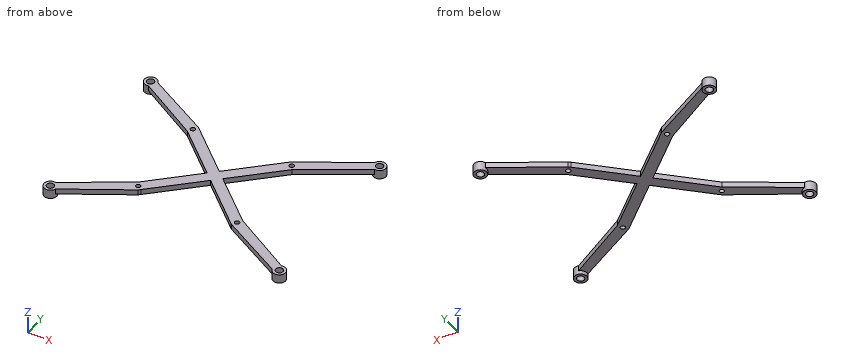
Autodesk Fusion 360 part; units mm, degrees
sketch "Sketch1" plane through (0, 0, 0) normal (0, 0, 1) x (1, 0, 0)
  line L0 (0, 0) -> (126.2, 0) construction
  line L1 (126.2, 0) -> (126.2, 92.7) construction
  line L2 (126.2, 92.7) -> (0, 92.7) construction
  line L3 (0, 92.7) -> (0, 0) construction
  circle A0 centre (126.2, 0) radius 2
  circle A1 centre (126.2, 92.7) radius 2
  circle A2 centre (0, 92.7) radius 2
  circle A3 centre (0, 0) radius 2
  line L4 (0, 92.7) -> (-5, 92.7) construction
  line L5 (0, 92.7) -> (0, 97.7) construction
  line L6 (0, 97.7) -> (-5, 92.7) construction
  line L7 (126.2, 0) -> (131.2, 0) construction
  line L8 (126.2, 0) -> (126.2, -5) construction
  line L9 (126.2, -5) -> (131.2, 0) construction
  line L10 (-2.5, 95.2) -> (128.7, 95.2)
  line L11 (128.7, 95.2) -> (128.7, -2.5)
  line L12 (128.7, -2.5) -> (-2.5, -2.5)
  line L13 (-2.5, -2.5) -> (-2.5, 95.2)
  line L14 (35.8499, 71.5999) -> (90.3499, 71.5999) construction
  line L15 (90.3499, 71.5999) -> (90.3499, 21.0999) construction
  line L16 (90.3499, 21.0999) -> (35.8499, 21.0999) construction
  line L17 (35.8499, 21.0999) -> (35.8499, 71.5999) construction
  line L18 (126.2, 0) -> (0, 92.7) construction
  line L19 (126.2, 92.7) -> (0, 0) construction
  line L20 (35.8499, 71.5999) -> (90.3499, 21.0999) construction
  line L21 (90.3499, 71.5999) -> (35.8499, 21.0999) construction
  circle A4 centre (35.8499, 71.5999) radius 1.3
  circle A5 centre (90.3499, 71.5999) radius 1.3
  circle A6 centre (90.3499, 21.0999) radius 1.3
  circle A7 centre (35.8499, 21.0999) radius 1.3
  circle A8 centre (90.3499, 71.5999) radius 3
  circle A9 centre (35.8499, 71.5999) radius 3
  circle A10 centre (35.8499, 21.0999) radius 3
  circle A11 centre (90.3499, 21.0999) radius 3
  circle A12 centre (126.2, 0) radius 2.5
  circle A13 centre (126.2, 92.7) radius 2.5
  circle A14 centre (0, 92.7) radius 2.5
  circle A15 centre (0, 0) radius 2.5
  line L22 (-1.5, 2) -> (34.2965, 23.6664)
  line L23 (1.5, -2) -> (37.3392, 18.4957)
  line L24 (91.9033, 23.6664) -> (127.4939, 2.1391)
  line L25 (88.8606, 18.4957) -> (124.7009, -2.0006)
  line L26 (37.3392, 74.2041) -> (1.5012, 94.6991)
  line L27 (34.2965, 69.0334) -> (-1.2939, 90.5609)
  line L28 (91.9033, 69.0334) -> (127.4939, 90.5609)
  line L29 (88.8606, 74.2041) -> (124.6996, 94.6997)
  line L30 (37.3392, 18.4957) -> (91.9033, 69.0334)
  line L31 (34.2965, 23.6664) -> (88.8606, 74.2041)
  line L32 (34.2965, 69.0334) -> (88.309, 18.9011)
  line L33 (91.9033, 23.6664) -> (37.3392, 74.2041)
  circle A16 centre (0, 92.7) radius 3.5
  circle A17 centre (0, 0) radius 3.5
  circle A18 centre (126.2, 0) radius 3.5
  circle A19 centre (126.2, 92.7) radius 3.5
  point P0 (-2.5, 95.2)
  point P1 (128.7, -2.5)
  dimension "d1" = 126.2
  dimension "d2" = 92.7
  dimension "d3" = 4
  dimension "d4" = 4
  dimension "d5" = 4
  dimension "d6" = 4
  dimension "d7" = 5
  dimension "d8" = 5
  dimension "d9" = 5
  dimension "d10" = 5
  dimension "d11" = 54.5
  dimension "d12" = 50.5
  dimension "d13" = 2.6
  dimension "d14" = 2.6
  dimension "d15" = 2.6
  dimension "d16" = 2.6
  dimension "d17" = 6
  dimension "d18" = 6
  dimension "d19" = 6
  dimension "d20" = 6
  dimension "d25" = 7
  dimension "d26" = 7
  dimension "d27" = 7
  dimension "d28" = 7
extrude "Extrude1" add sketch "Sketch1" along normal blind 3 contours A14 | A14 L26 L27 A16 | A9 L26 L27 A16 | A13 | A8 L28 L29 A19 | A13 L28 L29 A19 | A9 L33 | A15 L22 | A15 L22 L23 A17 | A10 L22 L23 A17 | A9 L31 L32 L33 | A8 L31 | A10 L30 L31 L32 | A10 L30 | L30 L31 L32 L33 | A8 L30 L31 L33 | A11 L30 L32 L33 | A11 | A12 | A11 L24 L25 A18 | A12 L24 L25 A18 picked at (37.444, 73.3682) picked at (-1.1921, 1.9962) picked at (88.7557, 73.3682) picked at (37.444, 19.3316)
extrude "Extrude2" add sketch "Sketch1" along normal blind -2 and the other way blind -3 contours L10 A16 | L10 L13 A14 A16 | L13 A16 | L10 A14 L26 A16 | A14 | L13 A14 L27 A16 | A14 L26 L27 A16 | L10 A19 | L10 A13 L29 A19 | L13 A15 L22 A17 | L13 A17 | L10 L11 A13 A19 | A13 | A13 L28 L29 A19 | L12 L13 A15 A17 | A15 L22 | A15 L22 L23 A17 | L11 A19 | L11 A13 L28 A19 | L12 A15 L23 A17 | L12 A17 | L11 A18 | L11 A12 L24 A18 | L12 A12 L25 A18 | L12 A18 | A12 | L11 L12 A12 A18 | A12 L24 L25 A18 picked at (-1.1921, 1.9962)
thread "Thread1"
Part model, mm, in its own coordinate system. Round coordinates to 2 decimals unless told otherwise and drop trailing zeros. Order: outer loops, then holes, each group sorted by start corner. A loop starts at its lowest first (then second) coordinate and runs counter-clockwise, first axis right, second up. Notation, with made-up numbers: M 17.25,2.25 L 43.25,2.25 A31 cw 43.25,35.25 Z; hole C -16.5,8 d3. An arc over 180 degrees is marked long. Answer in a Markdown table with one row per item. Add a question column.
Q1. Wall check: L1, parallel to Y at x = 0, z = -0.5; L2, parallel to X at y = 1, z = -1.5; L3, parallel to Z at x = 42.5, y = 23.5. Give the ranges that are in metal, low to high. Write a range as from..to.
Q2. Cut at A-A on y = 13. Give the cut face in (x, z), and give its area (3 significant figures).
Q3. Pin check, flat tips, straight feed: pin 1 (2 mm diameter, centred on y = 30.5, z = 1, fed in from -X); pin 2 (1.5 mm diameter, centred on y = 67.5, z = 2, fed in from -X). Stop position of each tip, or through.
Q4. Cut at C-C on z = 1.7. Give the number of separate pieces and of enclosed holes in the cut face, and give its area (3 significant figures).
Q5. Cut at B-B on x = 116. Give the cut face in (y, z), and give its area (3 significant figures).
Established:
| question | item | result |
|---|---|---|
| 1 | L1 | y = -3.5..-2, 2..3.5, 89.2..90.7, 94.7..96.2 |
| 1 | L2 | x = -3.35..-1.73, 1.73..3.35, 122.85..124.47, 127.93..129.55 |
| 1 | L3 | z = 0..3 |
| 2 | outline | M 16.67,0 L 27.73,0 L 27.73,3 L 16.67,3 Z; M 98.47,0 L 109.54,0 L 109.54,3 L 98.47,3 Z |
| 2 | area | 66.4 mm2 |
| 3 | pin 1 | stops at x = 40.59 |
| 3 | pin 2 | stops at x = 35.14 |
| 4 | separate pieces | 1 |
| 4 | enclosed holes | 9 |
| 4 | area | 1,770 mm2 |
| 5 | outline | M 2.98,0 L 9.09,0 L 9.09,3 L 2.98,3 Z; M 83.61,0 L 89.72,0 L 89.72,3 L 83.61,3 Z |
| 5 | area | 36.7 mm2 |
